For this review, use the dimensioned drawing (mm, ordinates from the lowest corner) and the shaded views. Round coordinates to 2 decimals unless told otherwise and drop trailing zeros. Write each loop counter-clockwise with the first axis right and the second up, starting at its lowest first coordinate (ties: lowest second). Pieces come first, ordered by that corner, then holes. Notation, with made-up numbers: (35, 85) -> (69, 85) arc R20 cw to (69, 97) -> close; hole circle Ø9 at (-34, 62.5). An arc over 180 degrees is marked (long way). Answer as CSV lines item,"result". Start each with the question number.
Item 1: Take a section at B-B on x = 118. Give the boundary of the cut face in (y, z) (1 decimal).
Item 2: Take a section at C-C on z = 85.5. Give the boundary of the cut face in (x, y) (1 decimal).
Item 3: For pin 1 Ø1 at (y, z) = (1.5, 201) entering from -X; pin 2 Ø1 at (x, y) = (3.5, 2) entering from -Z; pin 3 Ø1 at (x, y) = (122, 1.5) entering from +Z (1 decimal); pin 4 Ø1.6 at (x, y) = (122, 1) entering from -Z (1 decimal), all flat-tipped, find the tip position at first contact; note any pin that passes through.
Item 4: Wall thickness on probe 1 along X at (y, z) = (1.25, 94.5) (1 decimal); probe 2 along Z at (x, y) = (126.5, 1.7) (1 decimal): over which ranges is each line inside the solid? List them lowest first. Write a range as from..to.
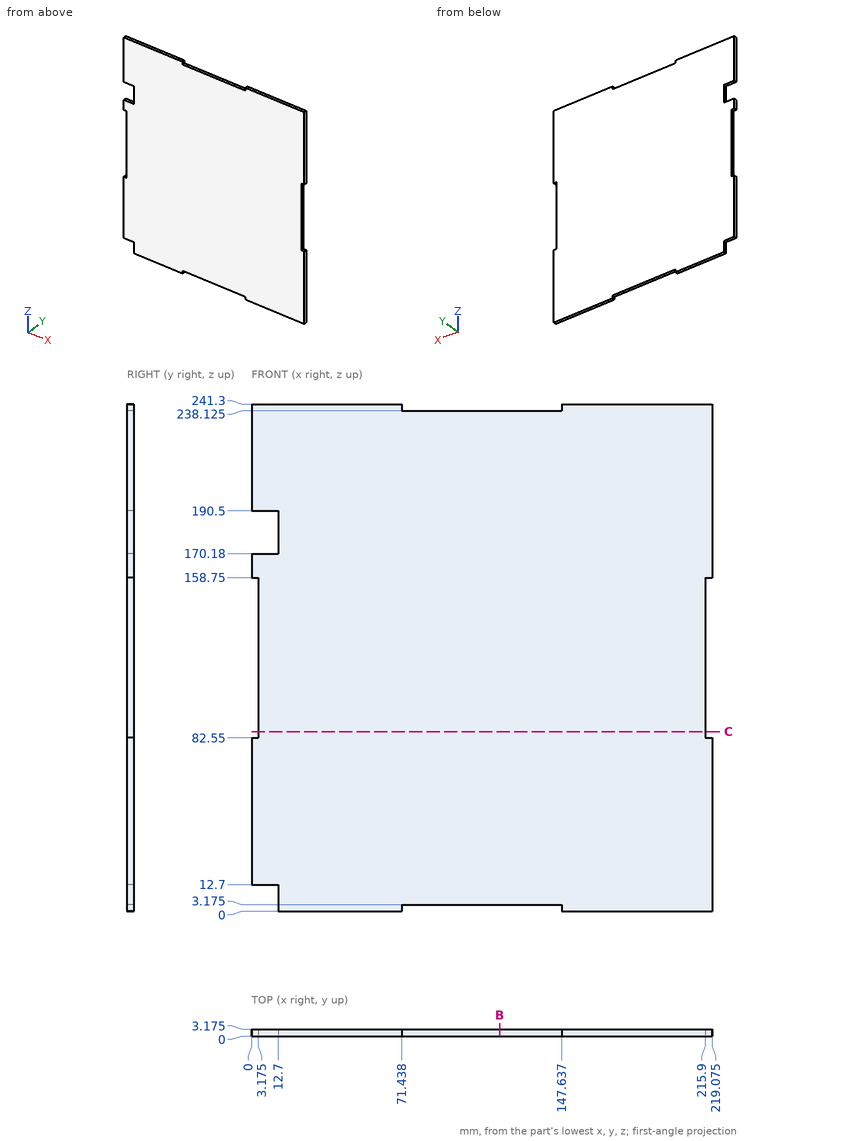
Output values:
1,outline,"(0, 3.2) -> (3.2, 3.2) -> (3.2, 238.1) -> (0, 238.1) -> close"
2,outline,"(3.2, 0) -> (215.9, 0) -> (215.9, 3.2) -> (3.2, 3.2) -> close"
3,pin 1,"stops at x = 0"
3,pin 2,"stops at z = 12.7"
3,pin 3,"stops at z = 238.1"
3,pin 4,"stops at z = 3.2"
4,probe 1,"x = 3.2..215.9"
4,probe 2,"z = 3.2..238.1"
